```python
from build123d import *

# Parameters (mm, degrees)
SKETCH1_W           = 63.5
SKETCH1_H           = 47.625
SKETCH1_R           = 8.89
SKETCH1_R_2         = 2.6543
SKETCH1_R_3         = 3.96875
BOSS_EXTRUDE1_DEPTH = 9.525
CUT_EXTRUDE2_START  = 5.55752
SKETCH1_3_R         = 8.89
SKETCH1_3_R_2       = 3.96875
CUT_EXTRUDE2_DEPTH  = 3.96748


with BuildPart() as part:
    # Sketch1 → Boss-Extrude1 (new body)
    # profile 1 of 3: a face of its own
    with BuildSketch(Plane.XY):
        with Locations((0, -23.8125)):
            Rectangle(SKETCH1_W, SKETCH1_H)
        with Locations((-15.875, -28.575)):
            Circle(SKETCH1_R, mode=Mode.SUBTRACT)
        with Locations(Location((11.1125, -4.7625, 0), (0, 0, 180))):
            Circle(SKETCH1_R_2, mode=Mode.SUBTRACT)
        with Locations(Location((-11.1125, -4.7625, 0), (0, 0, 180))):
            Circle(SKETCH1_R_2, mode=Mode.SUBTRACT)
        with Locations((15.875, -28.575)):
            Circle(SKETCH1_R, mode=Mode.SUBTRACT)
    # profile 2 of 3: a face of its own
    with BuildSketch(Plane.XY):
        with Locations((-15.875, -28.575)):
            Circle(SKETCH1_R)
        with Locations(Location((-15.875, -28.575, 0), (0, 0, 180))):
            Circle(SKETCH1_R_3, mode=Mode.SUBTRACT)
    # profile 3 of 3: a face of its own
    with BuildSketch(Plane.XY):
        with Locations((15.875, -28.575)):
            Circle(SKETCH1_R)
        with Locations(Location((15.875, -28.575, 0), (0, 0, 180))):
            Circle(SKETCH1_R_3, mode=Mode.SUBTRACT)
    extrude(amount=BOSS_EXTRUDE1_DEPTH)

    # Sketch1<3> → Cut-Extrude2 (cut)
    # profile 1 of 2: a face of its own
    with BuildSketch(Plane.XY.offset(CUT_EXTRUDE2_START)):
        with Locations((-15.875, -28.575)):
            Circle(SKETCH1_3_R)
        with Locations(Location((-15.875, -28.575, 0), (0, 0, 180))):
            Circle(SKETCH1_3_R_2, mode=Mode.SUBTRACT)
    # profile 2 of 2: a face of its own
    with BuildSketch(Plane.XY.offset(CUT_EXTRUDE2_START)):
        with Locations((15.875, -28.575)):
            Circle(SKETCH1_3_R)
        with Locations(Location((15.875, -28.575, 0), (0, 0, 180))):
            Circle(SKETCH1_3_R_2, mode=Mode.SUBTRACT)
    extrude(amount=CUT_EXTRUDE2_DEPTH, mode=Mode.SUBTRACT)


solid = part.part
```
Model file for the job. Use its own axes, mm. A direction names the side the tool comes from. Give positions to 0.01 mm unless a question says otherwise; leave off trailing zeros. Loops run counter-clockwise (first coordinate to the right, second up) from the corner with the lowest first, then second, coordinate; pieces in that order, holes last. Notation, with made-up numbers: (9, 33) -> (19, 33) arc R27 ccw to (19, 70) -> close; hole circle Ø3 at (66.5, 53). An arc over 180 degrees is marked (long way). Write each question's results on one line, items separated by ' | '.
(1) Pull direction Y, two halves, no side cores. Call faces 1 (the flat face through (0, -23, 0)), 2 (the flat face through (0, -47.625, 5)), 3 (the cylindrical face through (13.948, -37.254, 7.513)): released by +Y, released by -Y, zero draft, split by the parting line, or undercut.
Geometry results:
face 1: zero draft | face 2: released by -Y | face 3: undercut
(2) Cut at B-B on x = 18.5. List the corners of the cut face in (y, z) (3 decimals), and give its area (3 significant figures).
Geometry results:
outline: (-47.625, 0) -> (-31.552, 0) -> (-31.552, 5.558) -> (-37.069, 5.558) -> (-37.069, 9.525) -> (-47.625, 9.525) -> close; (-25.598, 0) -> (0, 0) -> (0, 9.525) -> (-20.081, 9.525) -> (-20.081, 5.558) -> (-25.598, 5.558) -> close | area: 353 mm²
(3) Cut at A-A on y = -25.5. List the corners of the cut face in (x, z) (3 decimals).
Geometry results:
outline: (-31.75, 0) -> (-18.384, 0) -> (-18.384, 5.558) -> (-24.216, 5.558) -> (-24.216, 9.525) -> (-31.75, 9.525) -> close; (-13.366, 0) -> (13.366, 0) -> (13.366, 5.558) -> (7.534, 5.558) -> (7.534, 9.525) -> (-7.534, 9.525) -> (-7.534, 5.558) -> (-13.366, 5.558) -> close; (18.384, 0) -> (31.75, 0) -> (31.75, 9.525) -> (24.216, 9.525) -> (24.216, 5.558) -> (18.384, 5.558) -> close
(4) Probe line 1 along Y through (x, z) = (11, 8) (3 decimals); line 2 along Y through (x, z) = (16, 2.25) (3 decimals); line 3 along X through (y, z) = (-7, 5.25). List the from-to ranges inside material, lowest first.
Geometry results:
line 1: y = -47.625 to -36.009, -21.141 to -7.414, -2.111 to 0 | line 2: y = -47.625 to -32.542, -24.608 to 0 | line 3: x = -31.75 to -12.54, -9.68 to 9.68, 12.54 to 31.75
(5) Cut at C-C on z = 7.5. Give the number of separate pieces and of enclosed holes in the cut face, and give its area (3 significant figures).
Geometry results:
separate pieces: 1 | enclosed holes: 4 | area: 2,480 mm²
(6) Cut at D-D on x = -22. List the corners of the cut face in (y, z) (3 decimals), and give its area (4 significant figures).
Geometry results:
outline: (-47.625, 0) -> (0, 0) -> (0, 9.525) -> (-22.132, 9.525) -> (-22.132, 5.558) -> (-35.018, 5.558) -> (-35.018, 9.525) -> (-47.625, 9.525) -> close | area: 402.5 mm²
(7) Flat gauge pins, fed straight in: pin 1 Ø19.5 at (x, y) = (-13.5, -32) entering from +Z (3 decimals); pin 2 Ø6.5 at (x, y) = (-15.875, -28.575) entering from +Z; pin 3 Ø1.5 at (x, y) = (12.5, -32.5) entering from +Z. Where does each tip first touch, or does it go through?
Geometry results:
pin 1: stops at z = 9.525 | pin 2: passes through | pin 3: stops at z = 5.56
(8) Tool access for faces 4 (the cylindrical face through (-7.663, -31.98, 7.513)), 5 (the cylindrical face through (8.58, -5.56, 4.7)): list every direction of +Z, -Z, +X, -X, +Y, -Y with a clear straight run to the whole face (end or side of a thin tool).
Geometry results:
face 4: +Z | face 5: +Z, -Z
